Work out the finished part from the listing and answer in its coordinate system (mm). A direction names the side the tool comes from. Coordinates: 2 decimals unless noted, no trailing zeros. Order: outer loops, then holes, each group sorted by start corner. A loop starts at its lowest first (then second) coordinate and runs counter-clockwise, first axis right, second up. Notation, with made-up numbers: M -7.5,7.5 L 21.5,7.5 A18 cw 21.5,36.5 Z; hole C 7,-5 d11. An arc over 180 degrees is marked long. Use a Markdown table: item, result. Add a question column.
from build123d import *

# Parameters (mm, degrees)
F1_DEPTH = 10


with BuildPart() as f1:
    # F0 (on Top) → F1 (new body)
    with BuildSketch(Plane.XY):
        Polygon((-24.450092, 18.142014), (-54.450092, 18.142014), (-47.450092, -21.857986), (-27.450092, -21.857986), (-20.450092, 18.142014), align=None)
        Polygon((-24.450092, 58.142014), (-54.450092, 18.142014), (-24.450092, 18.142014), align=None)
    extrude(amount=F1_DEPTH)


solid = f1.part
(1) Straight lines are drawn through the part: line 1 (Y direction, x = -38, z = 1.25); line 2 (X direction, y = 16, z = 6.5); line 3 (X direction, y = 7, z = 1.75). For each, find the intervals that lie inside material, in ascending order.
(2) A cutting plane is placed at C-C on y = 45. Write down the section's boundary in (x, z), plus the area to 3 significant figures.
(3) Given P1, Ø1.2, axis at x = -23, z = 5, coming from the +Y side; P2, Ø1.5, axis at y = -4.5, z = 3.5, coming from the -X side; P3, Ø1, axis at y = 23.5, z = 8.5, coming from the -X side, each flat-ended and moving along its own axis, determine where each tip first touches the part or whether it passes through.
(4) A cutting plane is placed at A-A on z = 4.25. Write down the section's boundary in (x, y), plus the area to 3 significant figures.
(5) A cutting plane is placed at B-B on x = -30. Write down the section's boundary in (y, z), plus the area to 3 significant figures.
(6) Which of the six approach directions +Z, -Z, +X, -X, +Y, -Y give full straight-line access (tool end or side, diameter ignored) to faces 1 (the flat face through (-39.24, 38.42, 4.93)), 2 (the flat face through (-24.45, 38, 5))?
From the geometry:
| question | item | result |
|---|---|---|
| 1 | line 1 | y = -21.86 to 40.08 |
| 1 | line 2 | x = -54.08 to -20.82 |
| 1 | line 3 | x = -52.5 to -22.4 |
| 2 | outline | M -34.31,0 L -24.45,0 L -24.45,10 L -34.31,10 Z |
| 2 | area | 98.6 mm2 |
| 3 | P1 | stops at y = 18.14 |
| 3 | P2 | stops at x = -50.62 |
| 3 | P3 | stops at x = -50.81 |
| 4 | outline | M -54.45,18.14 L -47.45,-21.86 L -27.45,-21.86 L -20.45,18.14 L -24.45,18.14 L -24.45,58.14 Z |
| 4 | area | 1,680 mm2 |
| 5 | outline | M -21.86,0 L 50.74,0 L 50.74,10 L -21.86,10 Z |
| 5 | area | 726 mm2 |
| 6 | face 1 | +Z, -Z, -X, +Y |
| 6 | face 2 | +Z, -Z, +X, +Y |
